Could you check a few things on this model? Use its own coordinates, in mm. Face numbers are marked on the shaded views. A direction names the side the tool comes from. Give positions to 0.01 mm unless a question says otherwise; leave off trailing zeros. Loops run counter-clockwise (first coordinate to the right, second up) from the corner with the lowest first, then second, coordinate; pieces in that order, holes last. Notation, with made-up numbers: (-8.75, 52) -> (-1.75, 52) arc R31 ccw to (-1.75, 91) -> close; hole circle Ø11 at (13.25, 67). An arc over 180 degrees is marked (long way). Write item = value, one per line. Start each with the question number.
1) I want a section at A-A (y = 0). List the corners of the cut face in (x, z) for me.
2) I want a section at B-B (x = 0). List the corners of the cut face in (y, z) for me, and give its area (3 significant figures).
3) On a 3-axis mill with a long thin cutter (end or side, diameter ignored), from which of +Z, -Z, +X, -X, +Y, -Y can I reach the whole of each face in a straight line? I mean the marked faces 1 and 2. Say none if no direction works.
4) I'm going to push flat-ended pins straight in: pin 1 Ø1.7 at (y, z) = (-21.5, 17.5) entering from +X; pin 2 Ø4 at (y, z) = (56, 19.5) entering from -X; pin 3 Ø8 at (x, z) = (35, 22) entering from +Y. Where does each tip first touch, or does it pass through?
5) I need wall thicknesses on probe 1 along Y at (x, z) = (-53.5, 22.75); probe 2 along Y at (x, z) = (-8, 28.75); probe 3 along X at (y, z) = (12.5, 8.5). Which ranges of each line are inside material? Lowest first, please. Write a range as from..to.
6) I want a section at C-C (y = -75.5). Count the separate pieces of the cut face and the enclosed holes in it, and give its area (3 significant figures).
7) If we mould it in two halves opening along X, with no side actions, what happens to the marked faces 3, 4 and 5? For each: +X half, -X half, draft (parallel to the pull), parting line (faces both ways), or undercut.
from build123d import *

# Parameters (mm, degrees)
SKETCH1_R           = 125
SKETCH1_R_2         = 20
BOSS_EXTRUDE1_DEPTH = 30
CUT_EXTRUDE1_REACH  = 181.304
SKETCH2_W           = 10
SKETCH2_H           = 10


with BuildPart() as part:
    # Sketch1 → Boss-Extrude1 (new body)
    with BuildSketch(Plane.XY):
        Circle(SKETCH1_R)
        Circle(SKETCH1_R_2, mode=Mode.SUBTRACT)
        with BuildLine():
            Line((-15, -45.82575695), (-15, -92.870878105))
            ThreePointArc((-15, -92.870878105), (-16.858595688, -96.760811131), (-21.052631579, -97.758819058))
            ThreePointArc((-21.052631579, -97.758819058), (-86.602540378, -50), (-95.187936538, 30.647295765))
            ThreePointArc((-95.187936538, 30.647295765), (-92.226618374, 33.780433428), (-87.928539711, 33.445057996))
            Line((-87.928539711, 33.445057996), (-47.186269666, 9.922497418))
            ThreePointArc((-47.186269666, 9.922497418), (-45.222911355, 7.845908192), (-44.717642699, 5.033133359))
            ThreePointArc((-44.717642699, 5.033133359), (-38.97114317, -22.5), (-18, -41.243181255))
            ThreePointArc((-18, -41.243181255), (-15.816699867, -43.087144162), (-15, -45.82575695))
        make_face(mode=Mode.SUBTRACT)
        with BuildLine():
            Line((15, -45.82575695), (15, -92.870878105))
            ThreePointArc((15, -92.870878105), (16.858595688, -96.760811131), (21.052631579, -97.758819058))
            ThreePointArc((21.052631579, -97.758819058), (86.602540378, -50), (95.187936538, 30.647295765))
            ThreePointArc((95.187936538, 30.647295765), (92.226618374, 33.780433428), (87.928539711, 33.445057996))
            Line((87.928539711, 33.445057996), (47.186269666, 9.922497418))
            ThreePointArc((47.186269666, 9.922497418), (45.222911355, 7.845908192), (44.717642699, 5.033133359))
            ThreePointArc((44.717642699, 5.033133359), (38.97114317, -22.5), (18, -41.243181255))
            ThreePointArc((18, -41.243181255), (15.816699867, -43.087144162), (15, -45.82575695))
        make_face(mode=Mode.SUBTRACT)
        with BuildLine():
            Line((-32.186269666, 35.903259532), (-72.928539711, 59.425820109))
            ThreePointArc((-72.928539711, 59.425820109), (-75.368022686, 62.980377703), (-74.135304959, 67.111523293))
            ThreePointArc((-74.135304959, 67.111523293), (0, 100), (74.135304959, 67.111523293))
            ThreePointArc((74.135304959, 67.111523293), (75.368022686, 62.980377703), (72.928539711, 59.425820109))
            Line((72.928539711, 59.425820109), (32.186269666, 35.903259532))
            ThreePointArc((32.186269666, 35.903259532), (29.406211487, 35.24123597), (26.717642699, 36.210047895))
            ThreePointArc((26.717642699, 36.210047895), (0, 45), (-26.717642699, 36.210047895))
            ThreePointArc((-26.717642699, 36.210047895), (-29.406211487, 35.24123597), (-32.186269666, 35.903259532))
        make_face(mode=Mode.SUBTRACT)
    extrude(amount=BOSS_EXTRUDE1_DEPTH)

    # Sketch2 → Cut-Extrude1 (cut, up to next)
    with BuildSketch(Plane.XY.offset(30), mode=Mode.PRIVATE) as cut_extrude1_sk1:
        with Locations((0, -20)):
            Rectangle(SKETCH2_W, SKETCH2_H)
    cut_extrude1_tool1 = extrude(cut_extrude1_sk1.sketch, amount=-CUT_EXTRUDE1_REACH, mode=Mode.PRIVATE) & part.part
    add(cut_extrude1_tool1.solids().sort_by_distance((0, -20, 30))[0], mode=Mode.SUBTRACT)

    # Sketch3 → Revolve-Thin1 (revolve)
    with BuildSketch(Plane(origin=(0, 0, 0), x_dir=(0, 0, -1), z_dir=(1, 0, 0)), mode=Mode.PRIVATE) as revolve_thin1_sk:
        Polygon((-30, 124.946096873), (-25, 124.946096873), (-15, 114.946096873), (-5, 124.946096873), (0, 124.946096873), (0, 134.946096873), (-9.142135624, 134.946096873), (-15, 129.088232497), (-20.857864376, 134.946096873), (-30, 134.946096873), align=None)
    revolve(revolve_thin1_sk.sketch.rotate(Axis((0, 0, -10.871805442), (0, 0, 1)), 90), axis=Axis((0, 0, -10.871805442), (0, 0, 1)))


solid = part.part
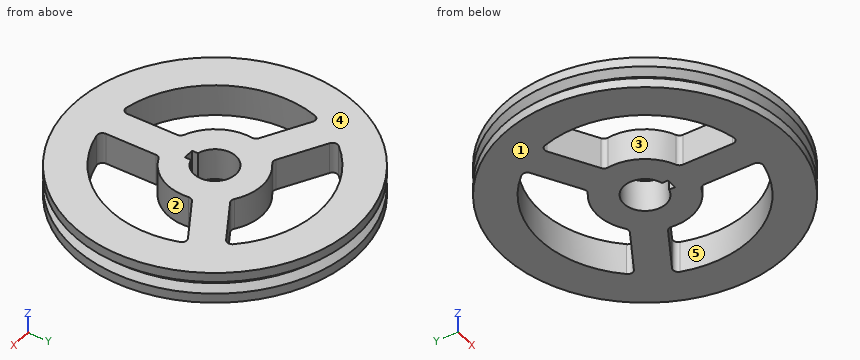
Answer list:
q1.outline = (-134.95, 0) -> (-100, 0) -> (-100, 30) -> (-134.95, 30) -> (-134.95, 20.86) -> (-129.09, 15) -> (-134.95, 9.14) -> close; (-45, 0) -> (-20, 0) -> (-20, 30) -> (-45, 30) -> close; (20, 0) -> (45, 0) -> (45, 30) -> (20, 30) -> close; (100, 0) -> (134.95, 0) -> (134.95, 9.14) -> (129.09, 15) -> (134.95, 20.86) -> (134.95, 30) -> (100, 30) -> close
q2.outline = (-134.95, 0) -> (-25, 0) -> (-25, 30) -> (-134.95, 30) -> (-134.95, 20.86) -> (-129.09, 15) -> (-134.95, 9.14) -> close; (20, 0) -> (45, 0) -> (45, 30) -> (20, 30) -> close; (100, 0) -> (134.95, 0) -> (134.95, 9.14) -> (129.09, 15) -> (134.95, 20.86) -> (134.95, 30) -> (100, 30) -> close
q2.area = 5,030 mm^2
q3.face_1 = -Z, +X, -X, +Y, -Y
q3.face_2 = +Z, -Z
q4.pin_1 = 130.69
q4.pin_2 = -123.44
q4.pin_3 = 131.34
q5.probe_1 = -123.89..-84.49, 13.57..48.21, 84.49..123.89
q5.probe_2 = -134.71..-18.33, 18.33..44.28, 99.68..134.71
q5.probe_3 = -134.37..-99.22, -51.65..-15.61, 15.61..51.65, 99.22..134.37
q6.separate_pieces = 3
q6.enclosed_holes = 0
q6.area = 3,590 mm^2
q7.face_3 = undercut
q7.face_4 = draft
q7.face_5 = undercut
